Read the model definition and answer for the solid it produces. Units are mm, in the model's axes. A direction names the side the tool comes from. Coordinates: 2 decimals unless noted, no trailing zeros. Order: outer loops, then holes, each group sorted by start corner. A loop starts at its lowest first (then second) coordinate and runs counter-clockwise, first axis right, second up. Notation, with made-up numbers: (8, 60) - (63, 60) arc R9 cw to (63, 72) - close; hole circle Ø9 at (12.25, -0.75). An arc over 180 degrees is marked (long way). Use one line per item in the form item = value.
```python
from build123d import *

# Parameters (mm, degrees)
SKETCH1_R           = 2.55
BASE_FLANGE1_DEPTH  = 1.2
BOSS_EXTRUDE1_DEPTH = 14
SKETCH11_W          = 1
SKETCH11_H          = 1.2
BOSS_EXTRUDE2_DEPTH = 14


# Sheet-metal steps are written as plain solids
with BuildPart() as part:
    # Sketch1 → Base-Flange1 (new body)
    with BuildSketch(Plane(origin=(0, 0, 0), x_dir=(1, 0, 0), z_dir=(0, 1, 0))):
        Polygon((0, 28), (0, 42), (-1, 42), (-1, 56), (0, 56), (0, 70), (15.75, 70), (15.75, 0), (0, 0), (0, 14), (-1, 14), (-1, 28), align=None)
        with Locations(Location((8.25, 62.5, 0), (0, 0, 270))):
            Circle(SKETCH1_R, mode=Mode.SUBTRACT)
        with Locations(Location((8.25, 35, 0), (0, 0, 270))):
            Circle(SKETCH1_R, mode=Mode.SUBTRACT)
        with Locations(Location((8.25, 7.5, 0), (0, 0, 270))):
            Circle(SKETCH1_R, mode=Mode.SUBTRACT)
    extrude(amount=-BASE_FLANGE1_DEPTH)

    # Sketch10 → Boss-Extrude1 (add)
    with BuildSketch(Plane.XY.offset(-42)):
        with BuildLine():
            Line((-3.25, -1.2), (-1, -1.2))
            Line((-1, -1.2), (0, -1.2))
            Line((0, -1.2), (0, 0))
            Line((0, 0), (-3.25, 0))
            ThreePointArc((-3.25, 0), (-4.699568901, 3.499568901), (-1.2, 2.05))
            Line((-1.2, 2.05), (-1.2, 0.145614193))
            Line((-1.2, 0.145614193), (0, 0.145614193))
            Line((0, 0.145614193), (0, 2.05))
            ThreePointArc((0, 2.05), (-5.548097039, 4.348097039), (-3.25, -1.2))
        make_face()
    extrude(amount=-BOSS_EXTRUDE1_DEPTH)

    # Sketch11 → Boss-Extrude2 (add)
    with BuildSketch(Plane.XY.offset(-14)):
        with BuildLine():
            ThreePointArc((-3.25, 0), (-4.699568901, 3.499568901), (-1.2, 2.05))
            Line((-1.2, 2.05), (-1.2, 0.145614193))
            Line((-1.2, 0.145614193), (0, 0.145614193))
            Line((0, 0.145614193), (-1.1e-07, 2.05))
            ThreePointArc((-1.1e-07, 2.05), (-5.548097133, 4.348096945), (-3.25, -1.2))
            Line((-3.25, -1.2), (-1, -1.2))
            Line((-1, -1.2), (-1, 0))
            Line((-1, 0), (-3.25, 0))
        make_face()
        with Locations((-0.5, -0.6)):
            Rectangle(SKETCH11_W, SKETCH11_H)
    extrude(amount=-BOSS_EXTRUDE2_DEPTH)


solid = part.part
```
(1) Section B-B, the plane x = 9.25 is taken. Write down the section's boundary in (y, z).
Answer list:
outline = (-1.2, -70) - (0, -70) - (0, -64.85) - (-1.2, -64.85) - close; (-1.2, -60.15) - (0, -60.15) - (0, -37.35) - (-1.2, -37.35) - close; (-1.2, -32.65) - (0, -32.65) - (0, -9.85) - (-1.2, -9.85) - close; (-1.2, -5.15) - (0, -5.15) - (0, 0) - (-1.2, 0) - close
(2) The mould has two halves that part along Y. Classify faces 1 (the cylindrical face through (-5.471, 4.423, -48.902)), 2 (the flat face through (4, -1.2, -35)), 3 (the flat face through (-1.2, 1, -49)): +Y half, -Y half, draft (parallel to the pull), parting line (faces both ways), or undercut.
Answer list:
face_1 = parting line
face_2 = -Y half
face_3 = undercut
(3) Straight lines are drawn through the part: L1, parallel to Y at x = -3.25, z = -48.75; L2, parallel to X at y = 2.05, z = -16.75; L3, parallel to Z at x = -1.5, y = -0.25. For each, find the intervals that lie inside material, in ascending order.
Answer list:
L1 = -1.2 to 0, 4.1 to 5.3
L2 = -6.5 to -5.3, -1.2 to 0
L3 = -56 to -42, -28 to -14
(4) Section D-D, the plane x = 1.25 is taken. Write down the section's boundary in (y, z).
Answer list:
outline = (-1.2, -70) - (0, -70) - (0, 0) - (-1.2, 0) - close
(5) Given pin 1 Ø8 at (x, z) = (9.5, -8.5) entering from +Y; pin 2 Ø0.6 at (y, z) = (-0.5, -34) entering from -X; pin 3 Ø1.9 at (x, y) = (-4, 3) entering from -Z; pin 4 Ø1 at (x, y) = (10.5, 1) entering from -Z, each flat-ended and moving along its own axis, determine where each tip first touches the part or whether it passes through.
Answer list:
pin_1 = 0
pin_2 = 0
pin_3 = -56
pin_4 = through
(6) Section C-C, the plane z = -55 is taken. Write down the section's boundary in (x, y).
Answer list:
outline = (-3.25, -1.2) - (15.75, -1.2) - (15.75, 0) - (-3.25, 0) arc R2.05 cw (long way) to (-1.2, 2.05) - (-1.2, 0.15) - (0, 0.15) - (0, 2.05) arc R3.25 ccw (long way) to start
(7) Section A-A, the plane z = -7.5 is taken. Write down the section's boundary in (x, y).
Answer list:
outline = (0, -1.2) - (5.7, -1.2) - (5.7, 0) - (0, 0) - close; (10.8, -1.2) - (15.75, -1.2) - (15.75, 0) - (10.8, 0) - close
(8) Which of the six approach directions +Z, -Z, +X, -X, +Y, -Y give full straight-line access (tool end or side, diameter ignored) to faces 4 (the flat face through (0, -1, -63)), 5 (the flat face through (-1.2, 1, -21)), 6 (the flat face through (-1, 2, -14))?
Answer list:
face_4 = -Z, -X, +Y, -Y
face_5 = +Z, -Z
face_6 = +Z, -X, +Y, -Y
